The figure shows three views and two pictorial views of one solid part (mm, origin at its lowest corner). Answer the questions. Coordinates: 2 decimals unless noted, no trailing zeros. Order: outer loops, then holes, each group sorted by start corner. A loop starts at its lowest first (then second) coordinate and runs counter-clockwise, first axis right, second up. Notation, with made-up numbers: (1.5, 31) -> (35.5, 31) arc R33 cw to (35.5, 59) -> close; hole circle Ø10 at (73.25, 13). An arc over 180 degrees is marked (long way). Return JSON: item names as keys, results as strings.
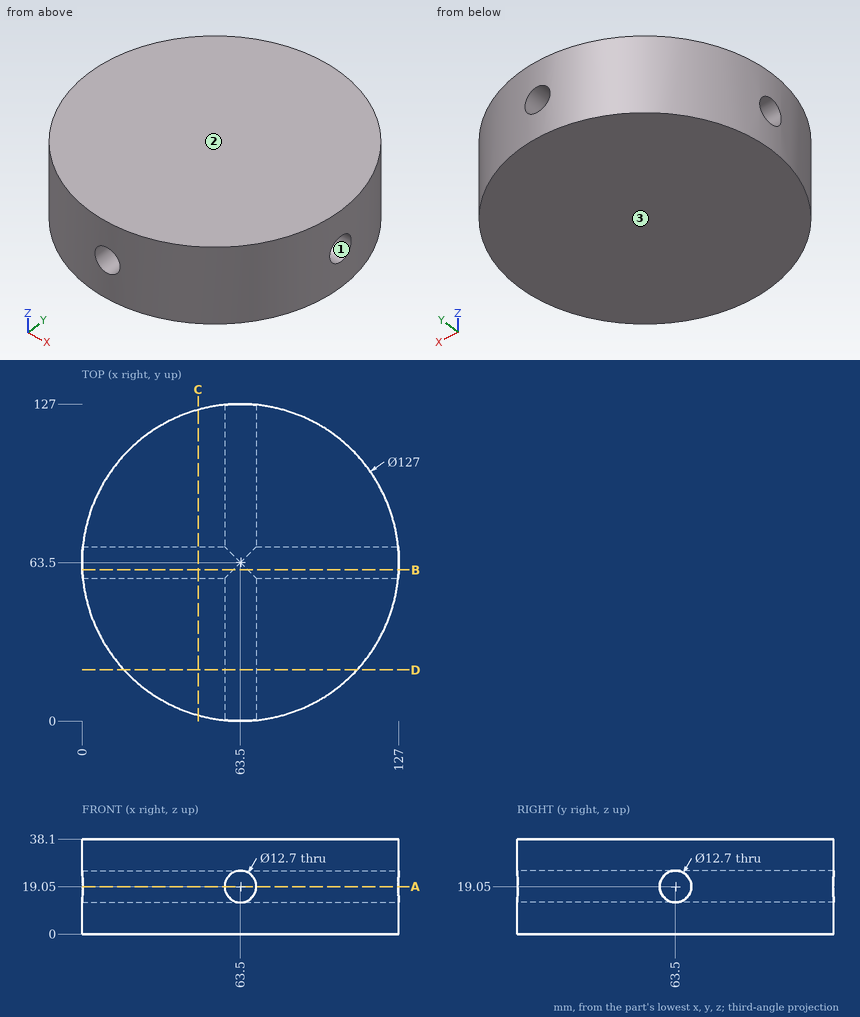
1. The part is cut by section D-D on y = 20.5. Give the vertices of the cut face in (x, z), and give its area (3 significant figures).
Answer block:
{"outline": "(16.77, 0) -> (110.23, 0) -> (110.23, 38.1) -> (16.77, 38.1) -> close; hole circle Ø12.7 at (63.5, 19.05)", "area": "3,430 mm2"}
2. The part is cut by section C-C on x = 46.5. Give the vertices of the cut face in (y, z), and give its area (3 significant figures).
Answer block:
{"outline": "(2.32, 0) -> (124.68, 0) -> (124.68, 38.1) -> (2.32, 38.1) -> close; hole circle Ø12.7 at (63.5, 19.05)", "area": "4,540 mm2"}
3. Determine the mould class of the marked faces 1, 2 and 3 for opening direction Z: pulls with the +Z half, pulls with the -Z half, needs draft (parallel to the pull), parting line crosses it, or undercut.
Answer block:
{"face 1": "undercut", "face 2": "pulls with the +Z half", "face 3": "pulls with the -Z half"}
4. The part is cut by section B-B on y = 60.5. Give the vertices of the cut face in (x, z), and give its area (3 significant figures).
Answer block:
{"outline": "(0.07, 0) -> (126.93, 0) -> (126.93, 13.45) -> (66.5, 13.45) arc R6.35 cw to (60.5, 13.45) -> (0.07, 13.45) -> close; (0.07, 24.65) -> (60.5, 24.65) arc R6.35 cw to (66.5, 24.65) -> (126.93, 24.65) -> (126.93, 38.1) -> (0.07, 38.1) -> close", "area": "3,410 mm2"}
5. The part is cut by section A-A on z = 19.05. Give the vertices of the cut face in (x, y), and give its area (3 significant figures).
Answer block:
{"outline": "(0.32, 57.15) arc R63.5 ccw to (57.15, 0.32) -> (57.15, 57.15) -> close; (0.32, 69.85) -> (57.15, 69.85) -> (57.15, 126.68) arc R63.5 ccw to start; (69.85, 0.32) arc R63.5 ccw to (126.68, 57.15) -> (69.85, 57.15) -> close; (69.85, 69.85) -> (126.68, 69.85) arc R63.5 ccw to (69.85, 126.68) -> close", "area": "9,610 mm2"}
6. Each of these flat-tipped pins is pushed along its axis until it touches: pin 1 Ø1 at (x, z) = (66.5, 33) entering from -Y; pin 2 Ø12 at (x, z) = (95.5, 5) entering from -Y; pin 3 Ø3 at (x, z) = (35, 21.5) entering from +Y. Where does it stop, or does it pass through?
Answer block:
{"pin 1": "stops at y = 0.05", "pin 2": "stops at y = 5.57", "pin 3": "stops at y = 120.97"}
7. Consider line 1 (Z direction, x = 77, y = 63); line 2 (X direction, y = 119, z = 17.5); line 3 (Y direction, x = 77.5, z = 23). Determine where each line is inside the solid, lowest interval first. Write a range as from..to.
Answer block:
{"line 1": "z = 0..12.72, 25.38..38.1", "line 2": "x = 32.65..57.34, 69.66..94.35", "line 3": "y = 1.56..58.53, 68.47..125.44"}
